Geometry check sheet. Reference: drawing and pictorial views, mm from the part's lowest x, y, z. A direction names the side the tool comes from. Round coordinates to 2 decimals unless told otherwise and drop trailing zeros. Loops run counter-clockwise (first coordinate to the right, second up) from the corner with the lowest first, then second, coordinate; pieces in that order, holes last. Notation, with made-up numbers: (63.25, 18.25) - (99.25, 18.25) arc R27 ccw to (99.25, 43.25) - close; hole circle Ø8 at (47, -25). An arc over 180 degrees is marked (long way). Answer as CSV lines item,"result". Start each with the question number.
1) Depth check by flat-ended pin: P1, Ø3, axis at y = 36, z = 7.5, coming from the -X side; P2, Ø4, axis at x = 24, z = 7.5, coming from the -Y side; P3, Ø3.5, axis at y = 35, z = 5, coming from the +X side; P4, Ø5, axis at y = 15, z = 5, coming from the +X side. Enter the tip coordinate at first touch or a pass-through.
2) Cross-section at A-A on x = 15. Record the boundary of the cut face in (y, z), and give its area (3 significant figures).
3) Access from +Z, -Z, +X, -X, +Y, -Y to the whole of each face (thin tool, end or side, straight path). Record for the marked faces 1, 2 and 3.
4) Cross-section at B-B on y = 35. Record the boundary of the cut face in (x, z), and give its area (3 significant figures).
5) Thickness scan on line 1 along Y through (x, z) = (21, 4.5); line 2 along Y through (x, z) = (15, 6.75); line 3 along X through (y, z) = (36.5, 1). Record the ranges inside material, lowest first.
6) Cross-section at C-C on y = 15. Record the boundary of the cut face in (x, z), and give its area (3 significant figures).
7) Cross-section at D-D on z = 5.75. Record the boundary of the cut face in (x, y), and give its area (3 significant figures).
8) Draft check along Z on the marked faces 4, 5, 6 and 7. Enter one of: released by +Z, released by -Z, zero draft, split by the parting line, or undercut.
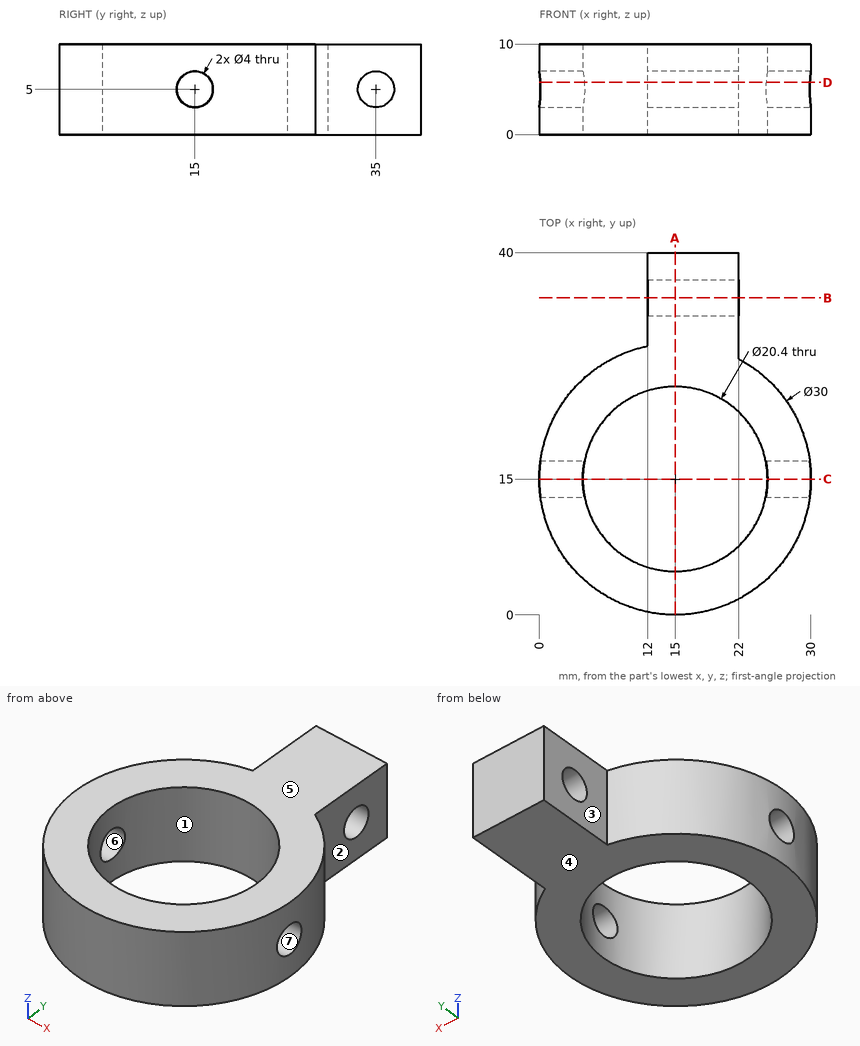
Answer block:
1,P1,"stops at x = 12"
1,P2,"stops at y = 1.73"
1,P3,"passes through"
1,P4,"stops at x = 30"
2,outline,"(0, 0) - (4.8, 0) - (4.8, 10) - (0, 10) - close; (25.2, 0) - (40, 0) - (40, 10) - (25.2, 10) - close; hole circle Ø4 at (35, 5)"
2,area,"183 mm^2"
3,face 1,"+Z, -Z"
3,face 2,"+Z, -Z, +X, +Y"
3,face 3,"+Z, -Z, -X, +Y"
4,outline,"(12, 0) - (22, 0) - (22, 3) - (12, 3) - close; (12, 7) - (22, 7) - (22, 10) - (12, 10) - close"
4,area,"60.0 mm^2"
5,line 1,"y = 1.25 to 6.75, 23.25 to 33.06, 36.94 to 40"
5,line 2,"y = 0 to 4.8, 25.2 to 34.03, 35.97 to 40"
5,line 3,"x = 12 to 22"
6,outline,"(0, 0) - (4.8, 0) - (4.8, 3) - (0, 3) - close; (0, 7) - (4.8, 7) - (4.8, 10) - (0, 10) - close; (25.2, 0) - (30, 0) - (30, 3) - (25.2, 3) - close; (25.2, 7) - (30, 7) - (30, 10) - (25.2, 10) - close"
6,area,"57.6 mm^2"
7,outline,"(0.12, 13.15) arc R15 ccw to (29.88, 13.15) - (25.03, 13.15) arc R10.2 cw to (4.97, 13.15) - close; (0.12, 16.85) - (4.97, 16.85) arc R10.2 cw to (25.03, 16.85) - (29.88, 16.85) arc R15 ccw to (22, 28.27) - (22, 33.15) - (12, 33.15) - (12, 29.7) arc R15 ccw to start; (12, 36.85) - (22, 36.85) - (22, 40) - (12, 40) - close"
7,area,"411 mm^2"
8,face 4,"released by -Z"
8,face 5,"released by +Z"
8,face 6,"undercut"
8,face 7,"undercut"
